Build history of the part. All positions in model axes, mm. A direction names the side the tool comes from. Give positions to 0.01 mm unless a question says otherwise; leave off trailing zeros. Order: outer loops, then holes, each group sorted by start corner. A loop starts at its lowest first (then second) coordinate and runs counter-clockwise, first axis right, second up. Notation, with made-up numbers: M 80,42.5 L 108,42.5 A29 ccw 108,76.5 Z; hole C 35,74.5 d8. An arc over 180 degrees is marked long. Answer as CSV lines item,"result".
from build123d import *

# Parameters (mm, degrees)
PAD_DEPTH       = 18
SKETCH001_R     = 3.3782
PAD001_DEPTH    = 4
SKETCH002_W     = 15
SKETCH002_H     = 25.4
POCKET_DEPTH    = 12
SKETCH003_R     = 3.61315
POCKET001_DEPTH = 6.215


with BuildPart() as part:
    # Sketch → Pad (new body)
    with BuildSketch(Plane.XY):
        with BuildLine():
            Line((-13.715, 10.7), (-13.715, -10.7))
            ThreePointArc((-13.715, -10.7), (-13.129214, -12.114214), (-11.715, -12.7))
            Line((-11.715, -12.7), (11.715, -12.7))
            ThreePointArc((11.715, -12.7), (13.129214, -12.114214), (13.715, -10.7))
            Line((13.715, -10.7), (13.715, 10.7))
            ThreePointArc((13.715, 10.7), (13.129214, 12.114214), (11.715, 12.7))
            Line((11.715, 12.7), (-11.715, 12.7))
            ThreePointArc((-11.715, 12.7), (-13.129214, 12.114214), (-13.715, 10.7))
        make_face()
    extrude(amount=PAD_DEPTH)

    # Sketch001 → Pad001 (join)
    with BuildSketch(Plane.XY):
        with BuildLine():
            Line((-33.8375, 10.7), (-33.8375, -10.7))
            ThreePointArc((-33.8375, -10.7), (-33.251714, -12.114214), (-31.8375, -12.7))
            Line((-31.8375, -12.7), (33.8375, -12.7))
            ThreePointArc((33.8375, -12.7), (35.251714, -12.114214), (35.8375, -10.7))
            Line((35.8375, -10.7), (35.8375, 10.7))
            ThreePointArc((35.8375, 10.7), (35.251714, 12.114214), (33.8375, 12.7))
            Line((33.8375, 12.7), (-31.8375, 12.7))
            ThreePointArc((-31.8375, 12.7), (-33.251714, 12.114214), (-33.8375, 10.7))
        make_face()
        with Locations((-25.4, 0)):
            Circle(SKETCH001_R, mode=Mode.SUBTRACT)
        with Locations((25.4, 0)):
            Circle(SKETCH001_R, mode=Mode.SUBTRACT)
    extrude(amount=-PAD001_DEPTH)

    # Sketch002 (on DatumPlane) → Pocket (cut)
    with BuildSketch(Plane.XY.offset(18)):
        Rectangle(SKETCH002_W, SKETCH002_H)
    extrude(amount=-POCKET_DEPTH, mode=Mode.SUBTRACT)

    # Sketch003 (on DatumPlane) → Pocket001 (cut)
    with BuildSketch(Plane.YZ.offset(13.715)):
        with Locations((0, 12)):
            Circle(SKETCH003_R)
    extrude(amount=-POCKET001_DEPTH, mode=Mode.SUBTRACT)


solid = part.part
Item 1: Band-saw the part on D-D (z = 12). Give the cut face in (x, y) (3 decimals), and give its area (3 significant figures).
Geometry says:
outline,"M -13.715,-10.7 A2 ccw -11.715,-12.7 L -7.5,-12.7 L -7.5,12.7 L -11.715,12.7 A2 ccw -13.715,10.7 Z; M 7.5,-12.7 L 11.715,-12.7 A2 ccw 13.715,-10.7 L 13.715,-3.613 L 7.5,-3.613 Z; M 7.5,3.613 L 13.715,3.613 L 13.715,10.7 A2 ccw 11.715,12.7 L 7.5,12.7 Z"
area,"267 mm2"
Item 2: Band-saw the part on B-B (x = -25.4). Give the cut face in (y, z), and give its area (3 significant figures).
Geometry says:
outline,"M -12.7,-4 L -3.38,-4 L -3.38,0 L -12.7,0 Z; M 3.38,-4 L 12.7,-4 L 12.7,0 L 3.38,0 Z"
area,"74.6 mm2"
Item 3: Pull direction X, two halves, no side cores. Call faces 1 (the flat face through (-13.715, 0, 9)), 2 (the cylindrical face through (22.025, 0.149, -1.972)), 3 (the flat face through (21, 0, 0)): released by +X, released by -X, zero draft, split by the parting line, or undercut.
Geometry says:
face 1,"released by -X"
face 2,"undercut"
face 3,"zero draft"
Item 4: Drop flat-ended pins along their axis: pin 1 (6 mm diameter, centred on y = -5, z = 11.5, fed in from +X) (3 decimals); pin 2 (4 mm diameter, centred on y = 10, z = 15.5, fed in from -X) (3 decimals); pin 3 (6.5 mm diameter, centred on y = 0, z = 12, fed in from +X); pin 4 (5.5 mm diameter, centred on x = 25.4, y = 0, fed in from -Z). Give the stop position or say it passes through.
Geometry says:
pin 1,"stops at x = 13.715"
pin 2,"stops at x = -13.715"
pin 3,"stops at x = -7.5"
pin 4,"passes through"
Item 5: Band-saw the part on C-C (y = 0). Give the cut face in (x, z) (1 decimal), and give its area (3 significant figures).
Geometry says:
outline,"M -33.8,-4 L -28.8,-4 L -28.8,0 L -33.8,0 Z; M -22,-4 L 22,-4 L 22,0 L 13.7,0 L 13.7,8.4 L 7.5,8.4 L 7.5,6 L -7.5,6 L -7.5,18 L -13.7,18 L -13.7,0 L -22,0 Z; M 7.5,15.6 L 13.7,15.6 L 13.7,18 L 7.5,18 Z; M 28.8,-4 L 35.8,-4 L 35.8,0 L 28.8,0 Z"
area,"493 mm2"
Item 6: Band-saw the part on A-A (z = -1.5). Give the cut face in (x, y).
Geometry says:
outline,"M -33.84,-10.7 A2 ccw -31.84,-12.7 L 33.84,-12.7 A2 ccw 35.84,-10.7 L 35.84,10.7 A2 ccw 33.84,12.7 L -31.84,12.7 A2 ccw -33.84,10.7 Z; hole C -25.4,0 d6.76; hole C 25.4,0 d6.76"
Item 7: 3-axis set-ups, long thin cutter, end or side, ignore diameter. For faces 4 (the cylindrical face through (-13.145, -12.099, 8.874)), 5 (the cylindrical face through (13.114, -12.13, 8.874)), 6 (the cylindrical face through (-13.114, 12.13, 8.874)), 7 (the cylindrical face through (10.7, -2.7, 14.4)): which of +Z, -Z, +X, -X, +Y, -Y reach the whole face in a straight line?
Geometry says:
face 4,"+Z, -X, -Y"
face 5,"+Z, +X, -Y"
face 6,"+Z, -X, +Y"
face 7,"+X"
Item 8: Probe line 1 along X through (y, z) = (-5.5, 7.25) (3 decimals); line 2 along Z through (x, y) = (12, 0); line 3 along Y through (x, z) = (-25.4, -1.4). List the from-to ranges inside material, lowest first. Write a range as from..to.
Geometry says:
line 1,"x = -13.715..-7.5, 7.5..13.715"
line 2,"z = -4..8.39, 15.61..18"
line 3,"y = -12.7..-3.38, 3.38..12.7"
